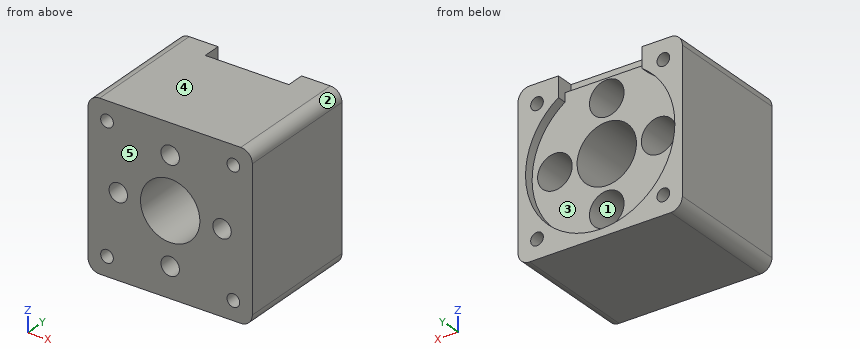
Autodesk Inventor part; units mm, degrees
ref_plane "YZ Plane" through (0, 0, 0) normal (1, 0, 0) x (0, 1, 0)
ref_plane "XZ Plane" through (0, 0, 0) normal (0, 1, 0) x (-1, 0, 0)
ref_plane "XY Plane" through (0, 0, 0) normal (0, 0, 1) x (1, 0, 0)
sketch "スケッチ4" plane through (0, 0, 0) normal (0, 1, 0) x (-1, 0, 0)
  line L0 (0, 0) -> (-28.5, 0)
  line L1 (-28.5, 0) -> (-28.5, -28.5)
  line L2 (-28.5, -28.5) -> (0, -28.5)
  line L3 (0, -28.5) -> (0, 0)
  dimension "d6" = 28.5
  dimension "d7" = 28.5
extrude "押し出し2" add sketch "スケッチ4" along normal blind 21.8
sketch "スケッチ5" plane through (0, 21.8, 0) normal (0, 1, 0) x (1, 0, 0)
  circle A0 centre (14.25, 14.25) radius 12.95
  line L0 (0, 28.5) -> (0, 0)
  line L1 (28.5, 28.5) -> (0, 28.5)
  line L2 (7, 3.5197) -> (21.5, 3.5197)
  line L3 (21.5, 3.5197) -> (21.5, -0.843)
  line L4 (21.5, -0.843) -> (7, -0.843)
  line L5 (7, -0.843) -> (7, 3.5197)
  point P0 (0, 14.25)
  point P1 (14.25, 28.5)
  point P2 (7, 1.3383)
  point P3 (21.5, 3.5197)
  dimension "d10" = 25.9
  dimension "d28" = 14.5
  dimension "d29" = 7.25
sketch "スケッチ6" plane through (0, 21.8, 0) normal (0, 1, 0) x (1, 0, 0)
  circle A0 centre (14.25, 14.25) radius 12.95
  line L0 (28.5, 0) -> (28.5, 28.5) construction
  line L1 (28.5, 28.5) -> (0, 28.5) construction
  line L2 (0, 0) -> (28.5, 0) construction
  circle A1 centre (24.5802, 2.4198) radius 0 construction
  circle A2 centre (14.25, 14.25) radius 15.5 construction
  line L3 (28.5, 0) -> (0, 28.5) construction
  line L4 (0, 28.5) -> (0, 0) construction
  line L5 (0, 0) -> (28.5, 28.5) construction
  point P0 (24.5802, 2.4198)
  point P1 (3.2898, 3.2898)
  point P2 (3.2898, 25.2102)
  point P3 (25.2102, 25.2102)
  point P4 (25.2102, 3.2898)
  dimension "d61" = 31
fillet "フィレット1" radius 2 4 edges at (0, 10.9, -28.5) (0, 10.9, 0) (28.5, 10.9, 0) (28.5, 10.9, -28.5)
extrude "押し出し3" cut sketch "スケッチ5" against normal blind 1.6
sketch "スケッチ7" plane through (0, 0, 0) normal (0, -1, 0) x (1, 0, 0)
  line L0 (0, -26.5) -> (0, -2)
  line L1 (26.5, -28.5) -> (2, -28.5)
  point P0 (0, 0)
  point P1 (14.25, -14.25)
  point P2 (0, -14.25)
  point P3 (14.25, -28.5)
hole "穴3" at (14.25, 0, -14.25) direction (0, 1, 0) diameter 10.3 end through all
sketch "スケッチ8" plane through (0, 0, 0) normal (0, -1, 0) x (1, 0, 0)
  line L0 (0, -26.5) -> (0, -2)
  line L1 (26.5, -28.5) -> (2, -28.5)
  circle A0 centre (14.25, -14.25) radius 9
  point P0 (0, 0)
  point P1 (0, -14.25)
  point P2 (14.25, -28.5)
  point P3 (14.25, -23.25)
  point P4 (5.25, -14.25)
  point P5 (14.25, -5.25)
  point P6 (23.25, -14.25)
  dimension "d39" = 18
hole "穴4" at (14.25, 0, -14.25) at (14.25, 0, -23.25) at (5.25, 0, -14.25) at (14.25, 0, -5.25) at (23.25, 0, -14.25) direction (0, 1, 0) diameter 3.2 end through all
sketch "スケッチ9" plane through (0, 20.2, 0) normal (0, 1, 0) x (1, 0, 0)
  circle A0 centre (14.25, 5.25) radius 1.6
  circle A1 centre (5.25, 14.25) radius 1.6
  circle A2 centre (14.25, 23.25) radius 1.6
  circle A3 centre (23.25, 14.25) radius 1.6
  point P0 (0, 0)
hole "穴5" at (14.25, 20.2, -5.25) at (5.25, 20.2, -14.25) at (14.25, 20.2, -23.25) at (23.25, 20.2, -14.25) direction (0, -1, 0) diameter 6 depth 15 tip angle 118
sketch "スケッチ10" plane through (0, 21.8, 0) normal (0, 1, 0) x (1, 0, 0)
  circle A0 centre (24.5802, 2.4198) radius 1.1
  circle A1 centre (2.4198, 2.4198) radius 1.1
  circle A2 centre (2.4198, 24.5802) radius 1.1
  circle A3 centre (24.5802, 24.5802) radius 1.1
  point P0 (0, 0)
hole "穴6" [suppressed]
hole "穴7" at (3.2898, 21.8, -3.2898) at (3.2898, 21.8, -25.2102) at (25.2102, 21.8, -25.2102) at (25.2102, 21.8, -3.2898) direction (0, -1, 0) diameter 2.2 end through all
sketch "スケッチ11" plane through (0, 20.2, 0) normal (0, 1, 0) x (1, 0, 0)
  line L0 (7, 0) -> (7, 3.5197)
  line L1 (21.5, 0) -> (7, 0)
  line L2 (7, 0) -> (7, 2)
  line L3 (7, 2) -> (21.5, 2)
  line L4 (21.5, 2) -> (21.5, 0)
  point P0 (7, 0)
  dimension "d72" = 2
extrude "押し出し5" cut sketch "スケッチ11" against normal blind 1.5
properties part number "NewPart1_for_shoulder"
Here's how the part is built. I have some questions about the finished solid (model axes, mm). Face numbers are marked on the shaded views. A direction names the side the tool comes from. Coordinates: 2 decimals unless noted, no trailing zeros. Order: outer loops, then holes, each group sorted by start corner. A loop starts at its lowest first (then second) coordinate and runs counter-clockwise, first axis right, second up.
1) I need wall thicknesses on line 1 (X direction, y = 7.5, z = -14.5); line 2 (X direction, y = 5.75, z = -11.5); line 3 (Z direction, x = 5.25, y = 14.5). Which ranges of each line are inside material? Lowest first, please.
2) Which directions (+Z, -Z, +X, -X, +Y, -Y) give clear straight access to the entire face, cutting with the end or side of a thin tool? Please do the marked faces 1 and 2.
3) Imagine slicing it at A-A on z = -14.25. List the corners of the cut face in (x, y) for me.
4) We'd pull the mould along Z, two halves only. Please class the marked faces 3, 4 and 5: +Z half, -Z half, draft (parallel to the pull), parting line (faces both ways), or undercut.
5) Imagine slicing it at B-B on x = 23.25. List the corners of the cut face in (y, z) for me, and give its area (3 significant figures).
6) Will these pins go through, and if not, where does the flat tip stop? pin 1 (7 mm diameter, centred on x = 14.25, z = -23.25, fed in from +Y); pin 2 (0.8 mm diameter, centred on x = 13.5, y = 19.5, fed in from +Z).
7) Imagine slicing it at D-D on y = 7.25. State how many separate pieces and enclosed holes the cut face has, and give its area (3 significant figures).
8) Imagine slicing it at C-C on z = -23.25. List the corners of the cut face in (x, y) for me.
Response values:
1. line 1: x = 0 to 2.26, 8.24 to 9.11, 19.39 to 20.26, 26.24 to 28.5
1. line 2: x = 0 to 4.05, 6.45 to 9.9, 18.6 to 22.05, 24.45 to 28.5
1. line 3: z = -28.5 to -17.25, -11.25 to 0
2. face 1: +Y
2. face 2: +Z, +X, +Y, -Y
3. outline: (0, 0) - (3.65, 0) - (3.65, 4.36) - (2.25, 5.2) - (2.25, 20.2) - (1.3, 20.2) - (1.3, 21.8) - (0, 21.8) - close; (6.85, 0) - (9.1, 0) - (9.1, 20.2) - (8.25, 20.2) - (8.25, 5.2) - (6.85, 4.36) - close; (19.4, 0) - (21.65, 0) - (21.65, 4.36) - (20.25, 5.2) - (20.25, 20.2) - (19.4, 20.2) - close; (24.85, 0) - (28.5, 0) - (28.5, 21.8) - (27.2, 21.8) - (27.2, 20.2) - (26.25, 20.2) - (26.25, 5.2) - (24.85, 4.36) - close
4. face 3: undercut
4. face 4: +Z half
4. face 5: draft
5. outline: (0, -28.5) - (21.8, -28.5) - (21.8, -23.56) - (20.2, -23.56) - (20.2, -17.25) - (5.2, -17.25) - (4.36, -15.85) - (0, -15.85) - close; (0, -12.65) - (4.36, -12.65) - (5.2, -11.25) - (20.2, -11.25) - (20.2, -4.94) - (21.8, -4.94) - (21.8, 0) - (0, 0) - close
5. area: 484 mm2
6. pin 1: stops at y = 20.2
6. pin 2: stops at z = -2
7. separate pieces: 1
7. enclosed holes: 9
7. area: 597 mm2
8. outline: (0, 0) - (12.65, 0) - (12.65, 4.36) - (11.25, 5.2) - (11.25, 20.2) - (4.94, 20.2) - (4.94, 21.8) - (0, 21.8) - close; (15.85, 0) - (28.5, 0) - (28.5, 21.8) - (23.56, 21.8) - (23.56, 20.2) - (17.25, 20.2) - (17.25, 5.2) - (15.85, 4.36) - close
